The model under review builds one solid part; all positions refer to its coordinate system, in mm. A direction names the side the tool comes from. Round coordinates to 2 decimals unless told otherwise and drop trailing zeros. Write each loop counter-clockwise with the first axis right and the second up, starting at its lowest first coordinate (ties: lowest second). Pieces come first, ordered by that corner, then holes. Notation, with made-up numbers: (72, 16) -> (125, 16) arc R30 cw to (125, 52) -> close; hole circle Ø1 at (64, 71). An arc over 180 degrees is marked (long way). Answer as a JSON object with one key per item and string values. Group by question number.
1) We need section A-A, the plane x = 0. Count the separate pieces of the cut face and the enclosed holes in it, then the cut area to 3 significant figures.
2) To check wall thickness, follow probe 1 along X at (y, z) = (9.5, 0); probe 2 along X at (y, z) = (14.5, -31.5); probe 3 along Z at (x, y) = (21, 15.5). State the ranges of each line that lie inside material, in increasing order. Write a range as [from, to].
3) Mouldability with a two-part tool opening along Z and no side actions: class faces 4 (the cylindrical face through (-9.912, 9.214, -31.476)), 5 (the flat face through (18, 12.7, -38)), 6 (the flat face through (18.215, 11.468, 40.91)), 7 (the cylindrical face through (21.063, 15.786, 30.973)) as pulls with the +Z half, pulls with the -Z half, needs draft (parallel to the pull), parting line crosses it, or undercut.
4) Machinability: for faces 1 (the flat face through (48, 3.2, -3)), 2 (the cylindrical face through (24, 16, -32)), 3 (the flat face through (-37.329, 15.996, -3.923)), which of the approach directions +Z, -Z, +X, -X, +Y, -Y give a long, thin tool a straight path to every point of the face, cutting with its end or side? Answer none if there is none.
5) Insertion check: pin 1 Ø1.5 at (x, z) = (-1.5, 35.5) entering from +Y; pin 2 Ø6 at (x, y) = (29.5, 4.5) entering from -Z; pin 3 Ø10 at (x, z) = (33, -6.5) entering from -Y; pin 4 Ø4.5 at (y, z) = (6.35, 0) entering from -X. Each pin has a flat end and moves straight along its axis. Give the tip position at first contact, or say it passes through.
6) We need section B-B, the plane y = 6. Write out the cut boundary in (x, z).
from build123d import *

# Parameters (mm, degrees)
SKETCH5_R          = 1.6425
CUT_EXTRUDE1_DEPTH = 50.7
SKETCH6_R          = 1.095
CUT_EXTRUDE2_DEPTH = 70.421071799
CIRPATTERN1_COUNT  = 4
CUT_EXTRUDE3_DEPTH = 6.5
CUT_EXTRUDE4_DEPTH = 2.5
CIRPATTERN2_COUNT  = 2
CIRPATTERN2_ANGLE  = 110
CIRPATTERN3_COUNT  = 2
CIRPATTERN3_ANGLE  = 110


with BuildPart() as part:
    # Sketch2 → Revolve1 (revolve)
    with BuildSketch(Plane.XY, mode=Mode.PRIVATE) as revolve1_sk:
        Polygon((49.7, 12.7), (49.7, 3.2004), (47.675, 3.2004), (47.675, 0), (44.7, 0), (33, 8.2), (33, 10.2), (35, 10.2), (35, 19.2), (40, 19.2), (40, 12.7), align=None)
    revolve(revolve1_sk.sketch.rotate(Axis((0, 0, 0), (0, 1, 0)), 90), axis=Axis((0, 0, 0), (0, 1, 0)))  # turned: the seam where the file's is

    # Sketch5 → Cut-Extrude1 (cut, through all)
    with BuildSketch(Plane.XY):
        with Locations(Location((0, 6.35, 0), (0, 0, 89.999999357))):  # turned: the seam where the file's is
            Circle(SKETCH5_R)
    cut_extrude1 = extrude(amount=-CUT_EXTRUDE1_DEPTH, mode=Mode.SUBTRACT)

    # Sketch6 → Cut-Extrude2 (cut, through all)
    with BuildSketch(Plane(origin=(0, 0, 0), x_dir=(0.809016994, 0, 0.587785252), z_dir=(-0.587785252, 0, 0.809016994))):
        with Locations((0, 14.7)):
            Circle(SKETCH6_R)
    cut_extrude2 = extrude(amount=-CUT_EXTRUDE2_DEPTH, mode=Mode.SUBTRACT)

    # CirPattern1: Cut-Extrude1 ×4 about axis
    cirpattern1_axis = Axis((0, 13.335, 0), (0, -1, 0))
    for i in range(1, CIRPATTERN1_COUNT):
        add(cut_extrude1.rotate(cirpattern1_axis, i * 360 / CIRPATTERN1_COUNT), mode=Mode.SUBTRACT)

    # Sketch7 → Cut-Extrude3 (cut)
    with BuildSketch(Plane(origin=(0, 19.2, 0), x_dir=(-1, 0, 0), z_dir=(0, 1, 0))):
        with BuildLine():
            Line((39.780875815, -4.181138531), (34.808266338, -3.658496214))
            ThreePointArc((34.808266338, -3.658496214), (20.57248383, 28.315594803), (-14.235782508, 31.974091017))
            Line((-14.235782508, 31.974091017), (-16.269465723, 36.541818306))
            ThreePointArc((-16.269465723, 36.541818306), (23.511410092, 32.360679775), (39.780875815, -4.181138531))
        make_face()
    extrude(amount=-CUT_EXTRUDE3_DEPTH, mode=Mode.SUBTRACT)

    # Sketch8 → Cut-Extrude4 (cut)
    with BuildSketch(Plane(origin=(0, 12.7, 0), x_dir=(1, 0, 0), z_dir=(0, 1, 0))):
        with BuildLine():
            Line((-49.4277382, 5.195064624), (-39.780875815, 4.181138531))
            ThreePointArc((-39.780875815, 4.181138531), (-23.511410092, -32.360679775), (16.269465723, -36.541818306))
            Line((16.269465723, -36.541818306), (20.214811161, -45.403209245))
            ThreePointArc((20.214811161, -45.403209245), (-29.212927039, -40.20814462), (-49.4277382, 5.195064624))
        make_face()
    extrude(amount=-CUT_EXTRUDE4_DEPTH, mode=Mode.SUBTRACT)

    # CirPattern2: Cut-Extrude2 ×2 about axis
    cirpattern2_axis = Axis((0, 13.335, 0), (0, -1, 0))
    for i in range(1, CIRPATTERN2_COUNT):
        add(cut_extrude2.rotate(cirpattern2_axis, i * CIRPATTERN2_ANGLE / (CIRPATTERN2_COUNT - 1)), mode=Mode.SUBTRACT)

    # CirPattern3: Cut-Extrude2 ×2 about axis
    cirpattern3_axis = Axis((0, 13.335, 0), (0, 1, 0))
    for i in range(1, CIRPATTERN3_COUNT):
        add(cut_extrude2.rotate(cirpattern3_axis, i * CIRPATTERN3_ANGLE / (CIRPATTERN3_COUNT - 1)), mode=Mode.SUBTRACT)


solid = part.part
Here are the results:
{
 "1": {"separate pieces": "4", "enclosed holes": "0", "area": "221 mm^2"},
 "2": {"probe 1": "x = [-49.7, -33], [33, 49.7]", "probe 2": "x = [-24.65, -15.26], [15.26, 21.56], [24.22, 24.65]", "probe 3": "z = [-34.04, -30.18], [28, 29.8], [32.47, 34.04]"},
 "3": {"face 4": "undercut", "face 5": "needs draft", "face 6": "pulls with the +Z half", "face 7": "undercut"},
 "4": {"face 1": "-Y", "face 2": "+Y", "face 3": "+Z, -X, +Y"},
 "5": {"pin 1": "stops at y = 12.7", "pin 2": "stops at z = -42.05", "pin 3": "stops at y = 4.25", "pin 4": "stops at x = -49.7"},
 "6": {"outline": "(-49.67, -1.6) arc R49.7 ccw to (-1.6, -49.67) -> (-1.6, -36.1) arc R36.14 cw to (-36.1, -1.6) -> close; (-49.67, 1.6) -> (-36.1, 1.6) arc R36.14 cw to (-1.6, 36.1) -> (-1.6, 49.67) arc R49.7 ccw to start; (1.6, -49.67) arc R49.7 ccw to (49.67, -1.6) -> (36.1, -1.6) arc R36.14 cw to (1.6, -36.1) -> close; (1.6, 36.1) arc R36.14 cw to (36.1, 1.6) -> (49.67, 1.6) arc R49.7 ccw to (1.6, 49.67) -> close"}
}
